Geometry check sheet. Reference: the model listing, model coordinates, mm. Face numbers are marked on the shaded views. A direction names the side the tool comes from. Give positions to 0.01 mm unless a question says otherwise; leave off trailing zeros. Write each loop counter-clockwise with the first axis right and the second up, starting at its lowest first coordinate (ties: lowest second). Pieces come first, ordered by that corner, then holes. Notation, with made-up numbers: M -36.75,42 L -30.75,42 A32 cw -30.75,78 Z; hole C 64.5,61.25 d4. An arc over 180 degrees is marked long. One line per item, written item: value. Start each with the question number.
1. Cross-section at A-A on z = -26. Record the cut outline in (x, y) (3 decimals), then the cut area to 3 significant figures.
2. Scan lines: line 1 (X direction, y = 10, z = 12); line 2 (Z direction, x = 67, y = 19.5); line 3 (X direction, y = 49.5, z = 33). Record each from-to range of solid material in increasing order.
3. Cross-section at D-D on x = 14. Record the cut outline in (y, z) (3 decimals).
4. Gauge pin test, flat ends, axial feed: pin 1 (6 mm diameter, centred on x = 33, y = 73, fed in from -Z); pin 2 (5 mm diameter, centred on y = 14.5, z = 13, fed in from -X) (3 decimals); pin 3 (9.5 mm diameter, centred on x = 29, z = 90, fed in from +Y). Record the tip position at first contact, or that the pin passes through.
5. Cross-section at B-B on y = 20.5. Count the separate pieces of the cut face and the enclosed holes in it, then the cut area to 3 significant figures.
6. Release check for a two-part mould opening along Z. For the marked faces 1, 2, 3 and 4 record: pulls with the +Z half, pulls with the -Z half, needs draft (parallel to the pull), parting line crosses it, or undercut.
7. Tool access check on the marked faces 5, 6 and 7. Record the directions out of +Z, -Z, +X, -X, +Y, -Y that give a thin tool (end or side, any length) a straight path to the whole face; none if there is none.
from build123d import *

# Parameters (mm, degrees)
BOSS_EXTRUDE1_DEPTH     = 2.54
SKETCH1_9_W             = 71.12
SKETCH1_9_H             = 71.12
BOSS_EXTRUDE3_DEPTH     = 63.5
SKETCH5_W               = 76.2
SKETCH5_H               = 76.2
SKETCH5_W_2             = 71.12
SKETCH5_H_2             = 71.12
BOSS_EXTRUDE4_DEPTH     = 25.4
BOSS_EXTRUDE7_DEPTH     = 19.05
BOSS_EXTRUDE11_DEPTH    = 19.05
SKETCH15_W              = 19.05
SKETCH15_H              = 6.35
BOSS_EXTRUDE12_DEPTH    = 19.05
SKETCH16_W              = 1.27
SKETCH16_H              = 12.7
CUT_EXTRUDE1_DEPTH      = 151.937776915
SKETCH17_W              = 6.35
SKETCH17_H              = 6.35
CUT_EXTRUDE2_DEPTH      = 25.4
CUT_EXTRUDE3_DEPTH      = 151.937776915
CUT_EXTRUDE3_DEPTH_BACK = 17.018
CUT_EXTRUDE4_DEPTH      = 162.394965845
CUT_EXTRUDE4_DEPTH_BACK = 12.7
SKETCH20_W              = 12.7
SKETCH20_H              = 2.54


with BuildPart() as part:
    # Sketch1 → Boss-Extrude1 (new body)
    with BuildSketch(Plane(origin=(0, 0, 0), x_dir=(1, 0, 0), z_dir=(0, 1, 0))):
        Polygon((-73.66, 73.66), (-73.66, -2.54), (0, -2.54), (0, -76.2), (76.2, -76.2), (76.2, 0), (2.54, 0), (2.54, 73.66), align=None)
    extrude(amount=-BOSS_EXTRUDE1_DEPTH)

    # Sketch1<9> → Boss-Extrude3 (add)
    with BuildSketch(Plane(origin=(0, 0, 0), x_dir=(1, 0, 0), z_dir=(0, 1, 0))):
        Polygon((2.54, 73.66), (-73.66, 73.66), (-73.66, -2.54), (0, -2.54), (0, -76.2), (76.2, -76.2), (76.2, 0), (2.54, 0), align=None)
        with Locations((38.1, -38.1)):
            Rectangle(SKETCH1_9_W, SKETCH1_9_H, mode=Mode.SUBTRACT)
        with Locations((-35.56, 35.56)):
            Rectangle(SKETCH1_9_W, SKETCH1_9_H, mode=Mode.SUBTRACT)
    extrude(amount=BOSS_EXTRUDE3_DEPTH)

    # Sketch5 → Boss-Extrude4 (add)
    with BuildSketch(Plane(origin=(0, 63.5, 0), x_dir=(1, 0, 0), z_dir=(0, 1, 0))):
        with Locations((38.1, -38.1)):
            Rectangle(SKETCH5_W, SKETCH5_H)
        with Locations((38.1, -38.1)):
            Rectangle(SKETCH5_W_2, SKETCH5_H_2, mode=Mode.SUBTRACT)
    extrude(amount=BOSS_EXTRUDE4_DEPTH)

    # Sketch9 → Boss-Extrude7 (add)
    with BuildSketch(Plane.XY.offset(2.54)):
        Polygon((-73.66, 3.81), (-73.66, -2.54), (0, -2.54), (0, 29.21), (-19.05, 29.21), (-19.05, 22.86), (-32.7025, 22.86), (-32.7025, 16.51), (-46.355, 16.51), (-46.355, 10.16), (-60.0075, 10.16), (-60.0075, 3.81), align=None)
    extrude(amount=BOSS_EXTRUDE7_DEPTH)

    # Sketch11 → Boss-Extrude11 (add)
    with BuildSketch(Plane.ZY):
        Polygon((76.2, 29.21), (21.59, 29.21), (21.59, 0), (21.59, -2.54), (76.2, -2.54), (76.2, 0), align=None)
        Polygon((21.59, 35.56), (21.59, 29.21), (76.2, 29.21), (76.2, 48.26), (76.2, 54.61), (62.5475, 54.61), (62.5475, 48.26), (48.895, 48.26), (48.895, 41.91), (35.2425, 41.91), (35.2425, 35.56), align=None)
    extrude(amount=BOSS_EXTRUDE11_DEPTH)

    # Sketch15 → Boss-Extrude12 (add)
    with BuildSketch(Plane.XY.offset(76.2)):
        Polygon((0, 60.96), (76.2, 60.96), (76.2, 88.9), (57.15, 88.9), (57.15, 81.915), (38.1, 81.915), (38.1, 74.93), (19.05, 74.93), (19.05, 67.945), (0, 67.945), align=None)
        Polygon((-19.05, 54.61), (-19.05, -2.54), (76.2, -2.54), (76.2, 60.96), (0, 60.96), (0, 54.61), align=None)
        with Locations((-9.525, 57.785)):
            Rectangle(SKETCH15_W, SKETCH15_H)
    extrude(amount=BOSS_EXTRUDE12_DEPTH)

    # Sketch16 → Cut-Extrude1 (cut, through all)
    with BuildSketch(Plane(origin=(0, 0, 0), x_dir=(1, 0, 0), z_dir=(0, 1, 0))):
        with Locations((-41.91, 25.185614026)):
            Rectangle(SKETCH16_W, SKETCH16_H)
        with Locations((-41.91, 39.37)):
            Rectangle(SKETCH16_W, SKETCH16_H)
        with Locations((-36.195, 39.37)):
            Rectangle(SKETCH16_W, SKETCH16_H)
        with Locations((-30.48, 39.37)):
            Rectangle(SKETCH16_W, SKETCH16_H)
        with Locations((-36.195, 25.185614026)):
            Rectangle(SKETCH16_W, SKETCH16_H)
        with Locations((-30.48, 25.185614026)):
            Rectangle(SKETCH16_W, SKETCH16_H)
        with Locations((19.685, -37.465)):
            Rectangle(SKETCH16_W, SKETCH16_H)
        with Locations((25.4, -37.465)):
            Rectangle(SKETCH16_W, SKETCH16_H)
        with Locations((31.115, -37.465)):
            Rectangle(SKETCH16_W, SKETCH16_H)
        with Locations((45.085, -37.465)):
            Rectangle(SKETCH16_W, SKETCH16_H)
        with Locations((50.8, -37.465)):
            Rectangle(SKETCH16_W, SKETCH16_H)
        with Locations((56.515, -37.465)):
            Rectangle(SKETCH16_W, SKETCH16_H)
    extrude(amount=-CUT_EXTRUDE1_DEPTH, mode=Mode.SUBTRACT)

    # Sketch17 → Cut-Extrude2 (cut)
    with BuildSketch(Plane.XZ.offset(2.54)):
        with Locations((-6.985, 12.065)):
            Rectangle(SKETCH17_W, SKETCH17_H)
        with Locations((-6.985, 85.725)):
            Rectangle(SKETCH17_W, SKETCH17_H)
        with Locations((66.675, 85.725)):
            Rectangle(SKETCH17_W, SKETCH17_H)
    extrude(amount=-CUT_EXTRUDE2_DEPTH, mode=Mode.SUBTRACT)

    # Sketch19 → Cut-Extrude3 (cut, two sides: drawn at the far end of the back side and taken through both)
    with BuildSketch(Plane.XY.offset(21.59).offset(-CUT_EXTRUDE3_DEPTH_BACK)):
        Polygon((-29.845, -312.284215123), (-29.845, -2.54), (-29.845, 0), (-42.545, 0), (-42.545, -2.54), (-42.545, -312.284215123), (-42.545, -931.77264537), (-29.845, -931.77264537), align=None)
    extrude(amount=CUT_EXTRUDE3_DEPTH + CUT_EXTRUDE3_DEPTH_BACK, mode=Mode.SUBTRACT)

    # Sketch20 → Cut-Extrude4 (cut, two sides: drawn at the far end of the back side and taken through both)
    with BuildSketch(Plane.ZY.offset(19.05).offset(-CUT_EXTRUDE4_DEPTH_BACK)):
        with Locations((37.465, -1.27)):
            Rectangle(SKETCH20_W, SKETCH20_H)
    extrude(amount=CUT_EXTRUDE4_DEPTH + CUT_EXTRUDE4_DEPTH_BACK, mode=Mode.SUBTRACT)


solid = part.part
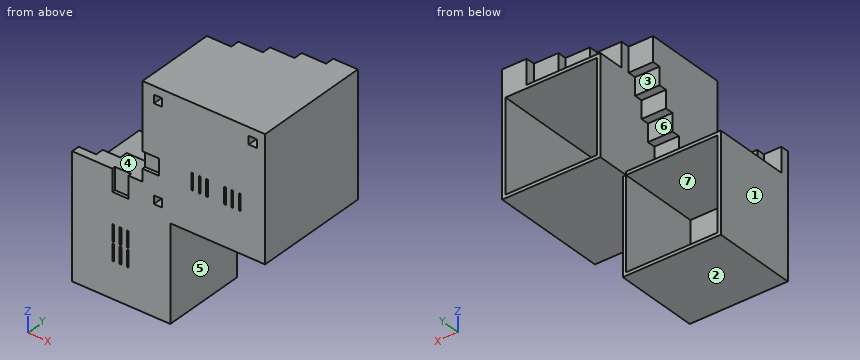
Report:
1. outline: M -73.66,-2.54 L -42.545,-2.54 L -42.545,0 L -71.12,0 L -71.12,63.5 L -73.66,63.5 Z; M -41.275,-2.54 L -36.83,-2.54 L -36.83,0 L -41.275,0 Z; M -35.56,-2.54 L -31.115,-2.54 L -31.115,0 L -35.56,0 Z; M -29.845,-2.54 L 2.54,-2.54 L 2.54,63.5 L 0,63.5 L 0,0 L -29.845,0 Z
1. area: 506 mm^2
2. line 1: x = -60.01 to -10.16, -3.81 to 2.54, 73.66 to 76.2
2. line 2: z = 0 to 2.54, 73.66 to 82.55, 88.9 to 95.25
2. line 3: x = 0 to 2.54, 73.66 to 76.2
3. outline: M -2.54,0 L 88.9,0 L 88.9,2.54 L 0,2.54 L 0,73.66 L 88.9,73.66 L 88.9,76.2 L 67.945,76.2 L 67.945,95.25 L -2.54,95.25 Z
4. pin 1: stops at z = 0
4. pin 2: stops at x = -46.355
4. pin 3: stops at y = 74.93
5. separate pieces: 1
5. enclosed holes: 5
5. area: 4,850 mm^2
6. face 1: needs draft
6. face 2: pulls with the -Z half
6. face 3: undercut
6. face 4: pulls with the +Z half
7. face 5: -Z, +X, +Y, -Y
7. face 6: -X, +Y
7. face 7: +Y
